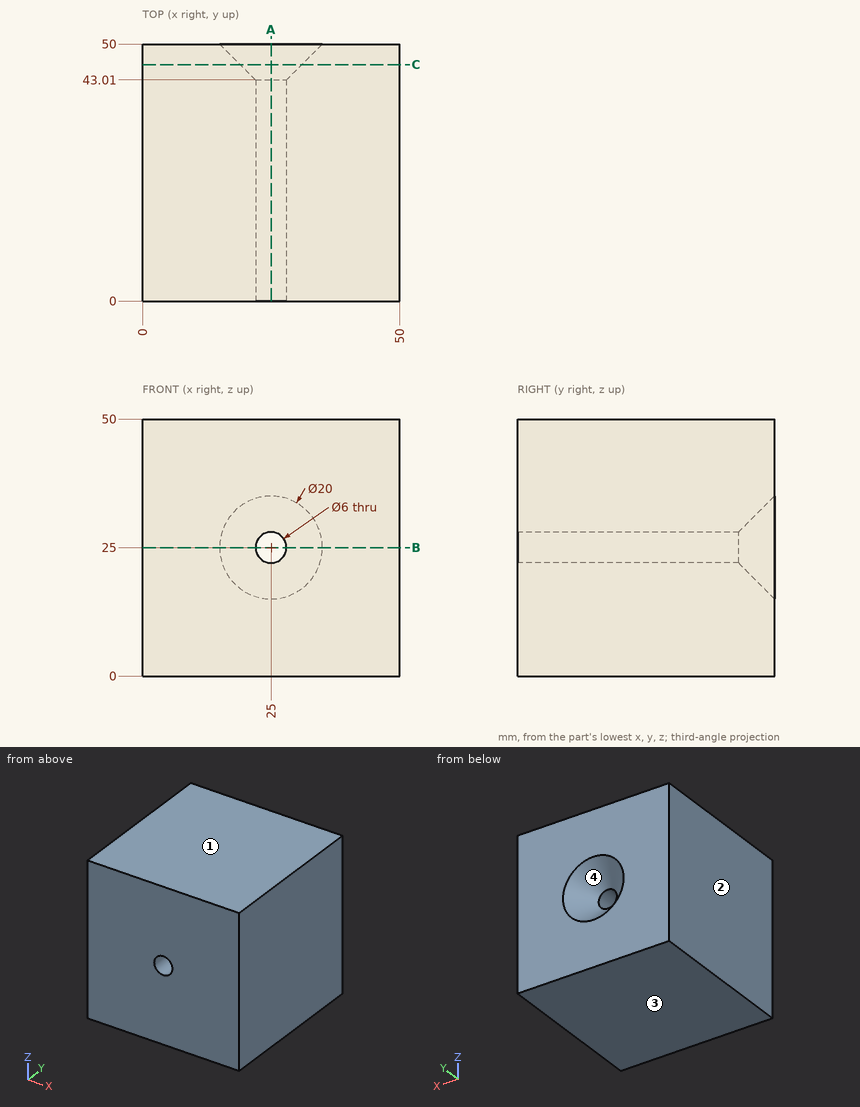
Can you work these out from the drawing? Everything is in mm from the part's minimum corner. Round coordinates to 2 decimals unless told otherwise and drop trailing zeros. Loops run counter-clockwise (first coordinate to the right, second up) from the corner with the lowest first, then second, coordinate; pieces in that order, holes last. Notation, with made-up numbers: (49.5, 80) - (62.5, 80) arc R14 ccw to (62.5, 85) - close; hole circle Ø3 at (-11.5, 64.5). An arc over 180 degrees is marked (long way). Answer in a Markdown table with one row per item. Add a question column.
Q1. I need wall thicknesses on L1, parallel to Z at x = 25, y = 16; L2, parallel to Z at x = 27.5, y = 15.5. Which ranges of each line are inside material? Lowest first, please.
Q2. I want a section at B-B on z = 25. List the corners of the cut face in (x, y) for me.
Q3. I want a section at C-C on y = 46. List the corners of the cut face in (x, z) for me, and give its area (3 significant figures).
Q4. For pin 1 Ø5.5 at (x, z) = (25, 25) entering from -Y, with a flat end and sliding along its axis, tell me the tip position at first contact or that it passes through.
Q5. I want a section at A-A on x = 25. List the corners of the cut face in (y, z) for me, and give its area (3 significant figures).
Q6. We'd pull the mould along Z, two halves only. Please class the marked faces 1, 2, 3 and 4: pulls with the +Z half, pulls with the -Z half, needs draft (parallel to the pull), parting line crosses it, or undercut.
A:
| question | item | result |
|---|---|---|
| 1 | L1 | 0 to 22, 28 to 50 |
| 1 | L2 | 0 to 23.34, 26.66 to 50 |
| 2 | outline | (0, 0) - (22, 0) - (22, 43.01) - (15, 50) - (0, 50) - close; (28, 0) - (50, 0) - (50, 50) - (35, 50) - (28, 43.01) - close |
| 3 | outline | (0, 0) - (50, 0) - (50, 50) - (0, 50) - close; hole circle Ø11.99 at (25, 25) |
| 3 | area | 2,390 mm^2 |
| 4 | pin 1 | through |
| 5 | outline | (0, 0) - (50, 0) - (50, 15) - (43.01, 22) - (0, 22) - close; (0, 28) - (43.01, 28) - (50, 35) - (50, 50) - (0, 50) - close |
| 5 | area | 2,150 mm^2 |
| 6 | face 1 | pulls with the +Z half |
| 6 | face 2 | needs draft |
| 6 | face 3 | pulls with the -Z half |
| 6 | face 4 | undercut |
